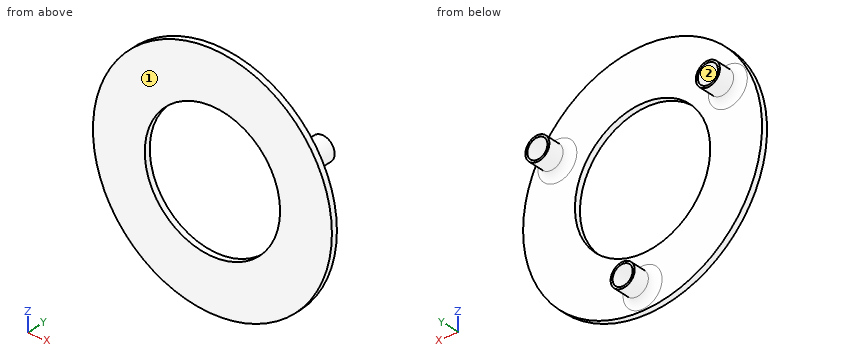
from build123d import *

# Parameters (mm, degrees)
SKETCH4_R           = 80
SKETCH4_R_2         = 45.315839153
BOSS_EXTRUDE1_DEPTH = 4
SKETCH4_3_R         = 8.046061865
SKETCH4_3_R_2       = 6.705051554
BOSS_EXTRUDE2_DEPTH = 20
FILLET1_R           = 5


with BuildPart() as part:
    # Sketch4 → Boss-Extrude1 (new body)
    with BuildSketch(Plane(origin=(0, 0, 0), x_dir=(1, 0, 0), z_dir=(0, 1, 0))):
        Circle(SKETCH4_R)
        Circle(SKETCH4_R_2, mode=Mode.SUBTRACT)
    extrude(amount=BOSS_EXTRUDE1_DEPTH)

    # Sketch4_3 → Boss-Extrude2 (add)
    with BuildSketch(Plane(origin=(0, 0, 0), x_dir=(1, 0, 0), z_dir=(0, 1, 0))):
        with Locations((-57.075283251, -32.954885136)):
            Circle(SKETCH4_3_R)
        with Locations((-57.075283251, -32.954885136)):
            Circle(SKETCH4_3_R_2, mode=Mode.SUBTRACT)
        with Locations((0.001262643, 65.904592273)):
            Circle(SKETCH4_3_R)
        with Locations((0.001262643, 65.904592273)):
            Circle(SKETCH4_3_R_2, mode=Mode.SUBTRACT)
        with Locations((57.077808537, -32.954885136)):
            Circle(SKETCH4_3_R)
        with Locations((57.077808537, -32.954885136)):
            Circle(SKETCH4_3_R_2, mode=Mode.SUBTRACT)
    extrude(amount=BOSS_EXTRUDE2_DEPTH)

    # Fillet1
    fillet1_edges = [part.edges().sort_by_distance(p)[0] for p in [
        (-65.121345116, 4, 32.954885136),
        (-8.044799222, 4, -65.904592273),
        (49.031746673, 4, 32.954885136),
    ]]
    fillet(fillet1_edges, radius=FILLET1_R)


solid = part.part
The model under review builds one solid part; all positions refer to its coordinate system, in mm. Face numbers are marked on the shaded views. Give positions to 0.01 mm unless a question says otherwise; leave off trailing zeros. Loops run counter-clockwise (first coordinate to the right, second up) from the corner with the lowest first, then second, coordinate; pieces in that order, holes last. Notation, with made-up numbers: (-11, 37) -> (31, 37) arc R25 ccw to (31, 49) -> close; hole circle Ø5 at (30.25, 6). An arc over 180 degrees is marked (long way). Answer as a JSON object with one key per item and string values. Group by question number.
Q1. Insertion check: pin 1 (6.5 mm diameter, centred on x = -54, z = 33, fed in from +Y); pin 2 (1 mm diameter, centred on x = -56.5, y = 8.5, fed in from -Z); pin 3 (5 mm diameter, centred on x = 53.5, z = 46.5, fed in from +Y). Each pin has a flat end and moves straight along its axis. Give the tip position at first contact, or say it passes through.
Q2. Take a section at A-A (z = 0). Write out the cut boundary in (x, y), plus the area to 3 significant figures.
Q3. Take a section at C-C (y = 2). Write out the cut boundary in (x, z), plus the area to 3 significant figures.
Q4. Wall thickness on line 1 along Z through (x, y) = (0, 1.3); line 2 along X through (y, z) = (10.5, 36); line 3 along X through (y, z) = (7, 35): over which ranges is each line inside the solid? List them lowest first.
Q5. Take a section at B-B (x = 42). Write out the cut boundary in (y, z), plus the area to 3 significant figures.
Q6. Draft analysis for pull direction X (two halves, no side actions). For the marked faces 1 and 2, state which applies: pulls with the +X half, pulls with the -X half, needs draft (parallel to the pull), parting line crosses it, or undercut.
Answer below:
{
 "1": {"pin 1": "stops at y = 4", "pin 2": "stops at z = 24.82", "pin 3": "stops at y = 4.24"},
 "2": {"outline": "(-80, 0) -> (-45.32, 0) -> (-45.32, 4) -> (-80, 4) -> close; (45.32, 0) -> (80, 0) -> (80, 4) -> (45.32, 4) -> close", "area": "277 mm2"},
 "3": {"outline": "circle Ø160 at (0, 0); hole circle Ø90.63 at (0, 0)", "area": "13,700 mm2"},
 "4": {"line 1": "z = -80 to -45.32, 45.32 to 80", "line 2": "x = -64.52 to -63.05, -51.1 to -49.63, 49.63 to 51.1, 63.05 to 64.53", "line 3": "x = -65.29 to -63.46, -50.69 to -48.86, 48.87 to 50.69, 63.46 to 65.29"},
 "5": {"outline": "(0, -68.09) -> (4, -68.09) -> (4, -17.02) -> (0, -17.02) -> close; (0, 17.02) -> (4, 17.02) -> (4, 68.09) -> (0, 68.09) -> close", "area": "409 mm2"},
 "6": {"face 1": "needs draft", "face 2": "undercut"}
}
